The model under review builds one solid part; all positions refer to its coordinate system, in mm. Round coordinates to 2 decimals unless told otherwise and drop trailing zeros. Write each loop counter-clockwise with the first axis right and the second up, starting at its lowest first coordinate (ties: lowest second). Pieces come first, ordered by that corner, then holes. Notation, with made-up numbers: (60, -13.75) - (75, -13.75) arc R13 cw to (75, 6.25) - close; hole circle Ø11 at (58, 76). An arc over 180 degrees is marked (long way). Use one line per item in the form item = value.
from build123d import *

# Parameters (mm, degrees)
SKETCH1_W           = 6.85
SKETCH1_H           = 19.5
BOSS_EXTRUDE2_DEPTH = 1.35
SKETCH2_R           = 2.5
CUT_EXTRUDE1_DEPTH  = 1.35
SKETCH3_R           = 0.475
CUT_EXTRUDE2_DEPTH  = 1.35


with BuildPart() as part:
    # Sketch1 → Boss-Extrude2 (new body)
    with BuildSketch(Plane(origin=(0, 0, 0), x_dir=(1, 0, 0), z_dir=(0, 1, 0))):
        with Locations((-0.149, 0)):
            Rectangle(SKETCH1_W, SKETCH1_H)
    extrude(amount=BOSS_EXTRUDE2_DEPTH)

    # Sketch2 → Cut-Extrude1 (cut)
    with BuildSketch(Plane.XZ):
        with Locations((0, -6.5)):
            Circle(SKETCH2_R)
    extrude(amount=-CUT_EXTRUDE1_DEPTH, mode=Mode.SUBTRACT)

    # Sketch3 → Cut-Extrude2 (cut)
    with BuildSketch(Plane(origin=(0, 1.35, 0), x_dir=(1, 0, 0), z_dir=(0, 1, 0))):
        with Locations((0, -7.87)):
            Circle(SKETCH3_R)
    extrude(amount=-CUT_EXTRUDE2_DEPTH, mode=Mode.SUBTRACT)


solid = part.part
(1) Add section D-D on x = 0. Write out the cut boundary in (y, z) (3 decimals), then the cut area to 3 significant figures.
Geometry results:
outline = (0, -9.75) - (1.35, -9.75) - (1.35, -9) - (0, -9) - close; (0, -4) - (1.35, -4) - (1.35, 7.395) - (0, 7.395) - close; (0, 8.345) - (1.35, 8.345) - (1.35, 9.75) - (0, 9.75) - close
area = 18.3 mm2
(2) Insertion check: P1, Ø4, axis at x = -1, z = -2, coming from the -Y side; P2, Ø3, axis at x = 0, z = -6.5, coming from the +Y side. Each pin has a flat end and moves straight along its axis. Give the tip position at first contact, or say it passes through.
Geometry results:
P1 = 0
P2 = through
(3) Add section C-C on y = 0.75. Write out the cut boundary in (x, z) (3 decimals), then the cut area to 3 significant figures.
Geometry results:
outline = (-3.574, -9.75) - (3.276, -9.75) - (3.276, 9.75) - (-3.574, 9.75) - close; hole circle Ø5 at (0, -6.5); hole circle Ø0.95 at (0, 7.87)
area = 113 mm2
(4) The part is to be moulded in two halves that separate along Z. For faces 1 (the cylindrical face through (-0.377, 0.684, 8.159)), 2 (the flat face through (0, 1.35, 2)), 3 (the flat face through (0, 1, -9.75)), 4 (the flat face through (0, 1, 9.75)), say which applies: +Z half, -Z half, draft (parallel to the pull), parting line (faces both ways), or undercut.
Geometry results:
face_1 = undercut
face_2 = draft
face_3 = -Z half
face_4 = +Z half
(5) Add section A-A on z = -4.5. Write out the cut boundary in (x, y).
Geometry results:
outline = (-3.57, 0) - (-1.5, 0) - (-1.5, 1.35) - (-3.57, 1.35) - close; (1.5, 0) - (3.28, 0) - (3.28, 1.35) - (1.5, 1.35) - close
(6) To check wall thickness, follow L1, parallel to Z at x = 0, y = 1.15 (3 decimals); L2, parallel to Z at x = 0.25, y = 0.7; L3, parallel to X at y = 0.35, z = 7.87 (3 decimals). State the ranges of each line that lie inside material, in increasing order.
Geometry results:
L1 = -9.75 to -9, -4 to 7.395, 8.345 to 9.75
L2 = -9.75 to -8.99, -4.01 to 7.47, 8.27 to 9.75
L3 = -3.574 to -0.475, 0.475 to 3.276
(7) Add section B-B on x = 2. Write out the cut boundary in (y, z).
Geometry results:
outline = (0, -9.75) - (1.35, -9.75) - (1.35, -8) - (0, -8) - close; (0, -5) - (1.35, -5) - (1.35, 9.75) - (0, 9.75) - close
